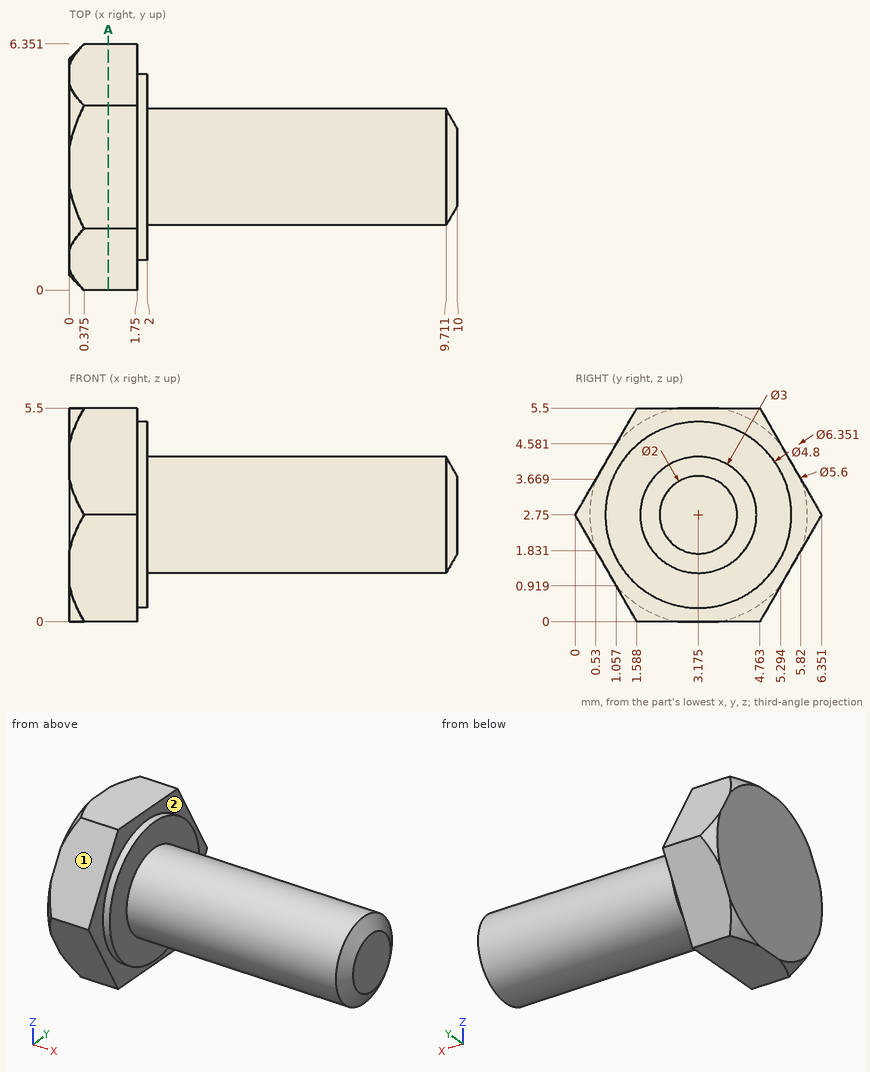
Answer from the drawing. Dimensions are ordinates in mm from the lowest x, y and z of the part. A direction names the side the tool comes from. Coordinates: 2 decimals unless noted, no trailing zeros. Order: outer loops, then holes, each group sorted by start corner. A loop starts at its lowest first (then second) coordinate and runs counter-clockwise, first axis right, second up. Notation, with made-up numbers: (-6, 1) - (45, 1) arc R23 ccw to (45, 36) - close; hole circle Ø4 at (8, 22.5). An arc over 180 degrees is marked (long way). Put each result on its own line as item: value. Start each with the question number.
1) Flat-ended cylindrical pins translate along their axes: pin 1 (1 mm diameter, centred on x = 8, y = 3.5, fed in from +Z); pin 2 (2 mm diameter, centred on x = 7, y = 4, fed in from -Z). Find the tip coordinate at first contact, or state that the pin passes through.
2) Find section A-A (x = 1). Give the vertices of the cut face in (y, z), plus the area to 3 significant figures.
3) Find the intervals of material crossed by line 1 (X direction, y = 4, z = 1.3); line 2 (X direction, y = 1, z = 4.4); line 3 (Z direction, x = 2.25, y = 3.25), in increasing order. Write a range as from..to.
4) For the marked faces 1 and 2, determine the directions among +Z, -Z, +X, -X, +Y, -Y from which every point of the face is accessible in a straight line to the end or side of a thin tool.
Results list:
1. pin 1: stops at z = 4.25
1. pin 2: stops at z = 1.25
2. outline: (0, 2.75) - (1.59, 0) - (4.76, 0) - (6.35, 2.75) - (4.76, 5.5) - (1.59, 5.5) - close
2. area: 26.2 mm^2
3. line 1: x = 0..2
3. line 2: x = 0..1.75
3. line 3: z = 1.25..4.25
4. face 1: +Z, +X, -X, -Y
4. face 2: +X
